Geometry check sheet. Reference: the model listing, model coordinates, mm. A direction names the side the tool comes from. Round coordinates to 2 decimals unless told otherwise and drop trailing zeros. Order: outer loops, then holes, each group sorted by start corner. A loop starts at its lowest first (then second) coordinate and runs counter-clockwise, first axis right, second up. Notation, with made-up numbers: (-22, 2) - (-16, 2) arc R18 cw to (-16, 6) - close; hole circle Ø4 at (79, 86.25). An arc over 180 degrees is marked (long way). Use a Markdown table: item, result. Add a question column.
(1) Access from +Z, -Z, +X, -X, +Y, -Y to the whole of each face (thin tool, end or side, straight path). Record for faces 1 (the face through (123, 0, -27)), 2 (the face through (112.86, -19.875, 11.577)), 3 (the face through (123, 0, 27)), 4 (the face through (252.748, -0.703, -15.985)).
(2) Section check A-A on y = -40. Record the boundary of the cut face in (x, z), then the cut area to 3 significant figures.
(3) Gauge pin test, flat ends, axial feed: P1, Ø2.5, axis at y = 0.5, z = -28.5, coming from the -X side; P2, Ø15.5, axis at y = 40, z = -25, coming from the +X side; P3, Ø6, axis at y = 5, z = -12.5, coming from the +X side; P4, Ø7, axis at y = 40, z = 25, coming from the +X side. Record the tip position at first contact, or that the pin passes through.
(4) Mould release check, pull along Z, two halves, no side actions. Record for faces 5 (the face through (138.07, -43.65, -20.24)), 6 (the face through (25.65, -12.65, 8.06)), 7 (the face through (364, -2, -11)): released by +Z, released by -Z, zero draft, split by the parting line, or undercut.
(5) Thickness scan on line 1 along Y through (x, z) = (141, -20); line 2 along Y through (x, z) = (142, -24.5); line 3 along X through (y, z) = (-34.5, 13). Record the ranges inside material, lowest first. Write a range as [from, to].
(6) Section check C-C on x = 327.5. Record the boundary of the cut face in (y, z), then the cut area to 3 significant figures.
(7) Section check B-B on x = 115. Record the boundary of the cut face in (y, z).
```python
from build123d import *

# Parameters (mm, degrees)
SKETCH_2_OUTSIDE_W       = 208.902
SKETCH_2_OUTSIDE_H       = 208.902
CUT_EXTRUDE_1_DEPTH      = 68
CUT_EXTRUDE_2_DEPTH      = 4
CUT_EXTRUDE_4_DEPTH      = 409.900966005
CUT_EXTRUDE_4_DEPTH_BACK = 409.900966005
SKETCH_6_R               = 3
SKETCH_7_R               = 6
CUT_EXTRUDE_5_DEPTH      = 271.645524626
SKETCH_8_OUTSIDE_W       = 208.902
SKETCH_8_OUTSIDE_H       = 208.902
SKETCH_8_OUTSIDE_W_2     = 80
SKETCH_8_OUTSIDE_H_2     = 120
CUT_EXTRUDE_6_DEPTH      = 271.645524626
CUT_EXTRUDE_3_DEPTH      = 20
PATTERN_CIRCULAR_1_COUNT = 6


with BuildPart() as part:
    # Эскиз1 → Повернуть1 (revolve)
    with BuildSketch(Plane.XY, mode=Mode.PRIVATE) as revolve_1_sk:
        with BuildLine():
            Line((129, 31), (103, 31))
            Line((103, 31), (103, 20))
            Line((103, 20), (51, 20))
            Line((51, 20), (51, 15))
            Line((51, 15), (1, 15))
            Line((1, 15), (0, 14))
            Line((0, 14), (0, 0))
            Line((0, 0), (400, 0))
            Line((400, 0), (400, 10.4))
            Line((400, 10.4), (398.4, 12))
            Line((398.4, 12), (370.1, 12))
            Line((370.1, 12), (368.146446609, 10.046446609))
            ThreePointArc((368.146446609, 10.046446609), (367.984234935, 9.938060234), (367.792893219, 9.9))
            Line((367.792893219, 9.9), (365, 9.9))
            ThreePointArc((365, 9.9), (364.292893219, 10.192893219), (364, 10.9))
            Line((364, 10.9), (364, 13.5))
            Line((364, 13.5), (361.5, 16))
            Line((361.5, 16), (147, 16))
            ThreePointArc((147, 16), (144.171572875, 17.171572875), (143, 20))
            Line((143, 20), (143, 60))
            Line((143, 60), (133, 60))
            Line((133, 60), (133, 35))
            ThreePointArc((133, 35), (131.828427125, 32.171572875), (129, 31))
        make_face()
    revolve(revolve_1_sk.sketch.rotate(Axis((0, 0, 0), (1, 0, 0)), 90), axis=Axis((0, 0, 0), (1, 0, 0)))

    # Эскиз2 outside → Вырез-Вытянуть1 (cut)
    with BuildSketch(Plane(origin=(400, 0, 0), x_dir=(0, 0, -1), z_dir=(1, 0, 0))):
        Rectangle(SKETCH_2_OUTSIDE_W, SKETCH_2_OUTSIDE_H)
        Polygon((0, -16.970562748), (16.970562748, 0), (0, 16.970562748), (-16.970562748, 0), align=None, mode=Mode.SUBTRACT)
    extrude(amount=-CUT_EXTRUDE_1_DEPTH, mode=Mode.SUBTRACT)

    # Эскиз3 → Вырез-Вытянуть2 (cut)
    with BuildSketch(Plane(origin=(0, 15, 0), x_dir=(1, 0, 0), z_dir=(0, 1, 0))):
        with BuildLine():
            Line((8, 4), (45, 4))
            ThreePointArc((45, 4), (49, 0), (45, -4))
            Line((45, -4), (8, -4))
            ThreePointArc((8, -4), (4, 0), (8, 4))
        make_face()
    extrude(amount=-CUT_EXTRUDE_2_DEPTH, mode=Mode.SUBTRACT)

    # Эскиз6 → Вырез-Вытянуть4 (cut, two sides: drawn at the far end of the back side and taken through both)
    with BuildSketch(Plane(origin=(0, 0, 0), x_dir=(1, 0, 0), z_dir=(0, 1, 0)).offset(-CUT_EXTRUDE_4_DEPTH_BACK)):
        with Locations(Location((392, 0, 0), (0, 0, 270))):
            Circle(SKETCH_6_R)
    extrude(amount=CUT_EXTRUDE_4_DEPTH + CUT_EXTRUDE_4_DEPTH_BACK, mode=Mode.SUBTRACT)

    # Эскиз7 → Вырез-Вытянуть5 (cut, through all)
    with BuildSketch(Plane(origin=(143, 0, 0), x_dir=(0, 0, -1), z_dir=(1, 0, 0))):
        with Locations((-25, 40)):
            Circle(SKETCH_7_R)
        with Locations((-25, -40)):
            Circle(SKETCH_7_R)
        with Locations((25, -40)):
            Circle(SKETCH_7_R)
        with Locations((25, 40)):
            Circle(SKETCH_7_R)
    extrude(amount=-CUT_EXTRUDE_5_DEPTH, mode=Mode.SUBTRACT)

    # Эскиз8 outside → Вырез-Вытянуть6 (cut, through all)
    with BuildSketch(Plane(origin=(143, 0, 0), x_dir=(0, 0, -1), z_dir=(1, 0, 0))):
        Rectangle(SKETCH_8_OUTSIDE_W, SKETCH_8_OUTSIDE_H)
        Rectangle(SKETCH_8_OUTSIDE_W_2, SKETCH_8_OUTSIDE_H_2, mode=Mode.SUBTRACT)
    extrude(amount=-CUT_EXTRUDE_6_DEPTH, mode=Mode.SUBTRACT)

    # Эскиз4 → Вырез-Вытянуть3 (cut)
    with BuildSketch(Plane.ZY.offset(-103)):
        with BuildLine():
            Line((30.740852298, 4), (27, 4))
            ThreePointArc((27, 4), (23, 0), (27, -4))
            Line((27, -4), (30.740852298, -4))
            ThreePointArc((30.740852298, -4), (31, 0), (30.740852298, 4))
        make_face()
    cut_extrude_3 = extrude(amount=-CUT_EXTRUDE_3_DEPTH, mode=Mode.SUBTRACT)

    # Круговой массив1: Вырез-Вытянуть3 ×6 about axis
    pattern_circular_1_axis = Axis((0, 0, 0), (1, 0, 0))
    for i in range(1, PATTERN_CIRCULAR_1_COUNT):
        add(cut_extrude_3.rotate(pattern_circular_1_axis, i * 360 / PATTERN_CIRCULAR_1_COUNT), mode=Mode.SUBTRACT)


solid = part.part
```
Check sheet entries:
| question | item | result |
|---|---|---|
| 1 | face 1 | -Z, -X |
| 1 | face 2 | -X |
| 1 | face 3 | +Z, -X |
| 1 | face 4 | +X |
| 2 | outline | (133, -40) - (143, -40) - (143, -31) - (133, -31) - close; (133, -19) - (143, -19) - (143, 19) - (133, 19) - close; (133, 31) - (143, 31) - (143, 40) - (133, 40) - close |
| 2 | area | 560 mm2 |
| 3 | P1 | stops at x = 123 |
| 3 | P2 | stops at x = 143 |
| 3 | P3 | stops at x = 399.94 |
| 3 | P4 | passes through |
| 4 | face 5 | undercut |
| 4 | face 6 | split by the parting line |
| 4 | face 7 | zero draft |
| 5 | line 1 | y = [-56.57, -43.32], [-36.68, 36.68], [43.32, 56.57] |
| 5 | line 2 | y = [-54.77, -45.98], [-34.02, 34.02], [45.98, 54.77] |
| 5 | line 3 | x = [133, 143] |
| 6 | outline | circle Ø32 at (0, 0) |
| 6 | area | 804 mm2 |
| 7 | outline | (-28.62, -11.91) - (-25.38, -10.04) arc R4 cw to (-21.38, -16.96) - (-24.62, -18.83) arc R31 ccw to (-4, -30.74) - (-4, -27) arc R4 cw to (4, -27) - (4, -30.74) arc R31 ccw to (24.62, -18.83) - (21.38, -16.96) arc R4 cw to (25.38, -10.04) - (28.62, -11.91) arc R31 ccw to (28.62, 11.91) - (25.38, 10.04) arc R4 cw to (21.38, 16.96) - (24.62, 18.83) arc R31 ccw to (4, 30.74) - (4, 27) arc R4 cw to (-4, 27) - (-4, 30.74) arc R31 ccw to (-24.62, 18.83) - (-21.38, 16.96) arc R4 cw to (-25.38, 10.04) - (-28.62, 11.91) arc R31 ccw to start |
